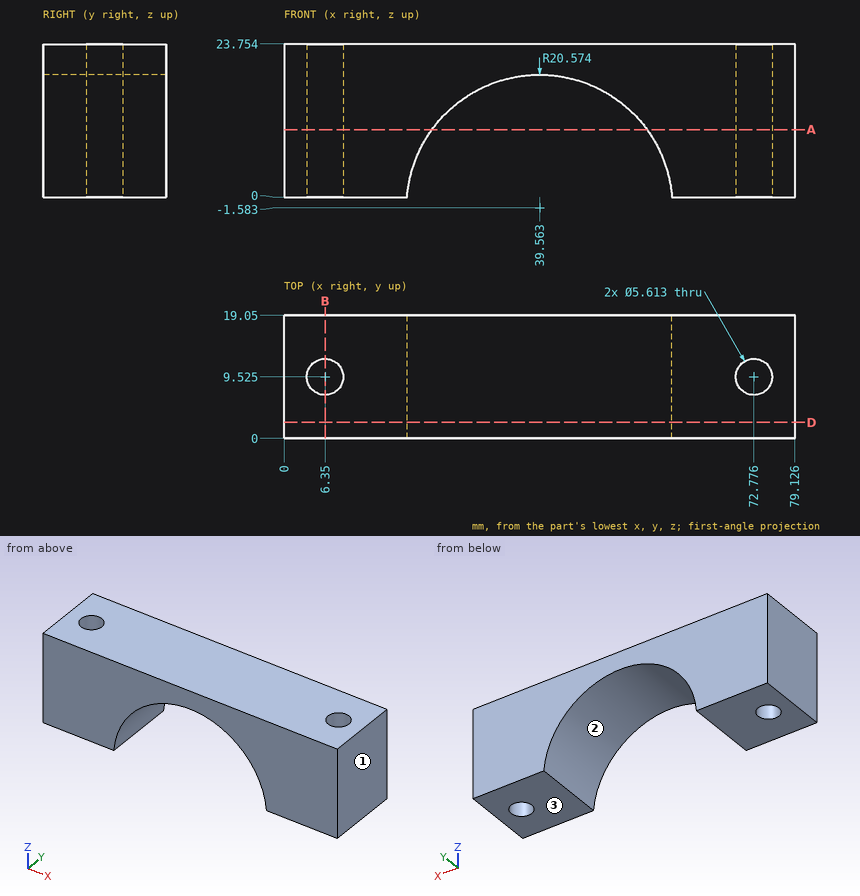
Here's the drawing with two shaded views (mm, measured from the low corner). I have some questions. Coordinates: 2 decimals unless noted, no trailing zeros. Write each loop counter-clockwise with the first axis right and the second up, starting at its lowest first coordinate (ties: lowest second). Pieces come first, ordered by that corner, then holes. Notation, with made-up numbers: (54.5, 6.5) -> (68.5, 6.5) arc R15 cw to (68.5, 17.5) -> close; hole circle Ø4 at (30, -39.5). An arc over 180 degrees is marked (long way). One line per question, with ' | ' between items. Start each with the question number.
1. Will these pins go through, and if not, where does the flat tip stop? P1, Ø10, axis at x = 47, z = 6.5, coming from the -Y side; P2, Ø10, axis at x = 50.5, y = 4.5, coming from the -Z side; P3, Ø5, axis at x = 25.5, y = 2, coming from the -Z side.
2. If we section it at A-A (z = 10.5): Count the separate pieces of the cut face and the enclosed holes in it.
3. If we section it at D-D (y = 2.5): Please give me the cut outline in (x, z).
4. Please list where these lines run through material, in increasing order: line 1 along Y through (x, z) = (6.35, 7.75); line 2 along X through (y, z) = (17, 3) (1 decimal); line 3 along X through (y, z) = (5, 14) (1 decimal).
5. Thinking about a two-plate mould opening in X: for the marked faces 1, 2 and 3, which applies, pulls with the +X half, pulls with the -X half, needs draft (parallel to the pull), parting line crosses it, or undercut?
6. If we section it at B-B (x = 6.35): Please give me the cut outline in (y, z).
Return value:
1) P1: passes through | P2: stops at z = 11.43 | P3: stops at z = 10.62
2) separate pieces: 2 | enclosed holes: 2
3) outline: (0, 0) -> (19.05, 0) arc R20.57 cw to (60.08, 0) -> (79.13, 0) -> (79.13, 23.75) -> (0, 23.75) -> close
4) line 1: y = 0 to 6.72, 12.33 to 19.05 | line 2: x = 0 to 19.5, 59.6 to 79.1 | line 3: x = 0 to 26.1, 53 to 79.1
5) face 1: pulls with the +X half | face 2: undercut | face 3: needs draft
6) outline: (0, 0) -> (6.72, 0) -> (6.72, 23.75) -> (0, 23.75) -> close; (12.33, 0) -> (19.05, 0) -> (19.05, 23.75) -> (12.33, 23.75) -> close
